Check sheet for the modelled part. Datum: model origin and axes. Units: mm. Face numbers are marked on the shaded views. A direction names the side the tool comes from. Give positions to 0.01 mm unless a question says otherwise; leave off trailing zeros. Order: outer loops, then holes, each group sorted by start corner. A loop starts at its lowest first (then second) coordinate and runs counter-clockwise, first axis right, second up. Notation, with made-up numbers: (-32.75, 76) -> (0.25, 76) arc R7 cw to (0.25, 87) -> close; hole circle Ø3 at (53, -22). An arc over 180 degrees is marked (long way). Write each question's results on one line, items separated by ' | '.
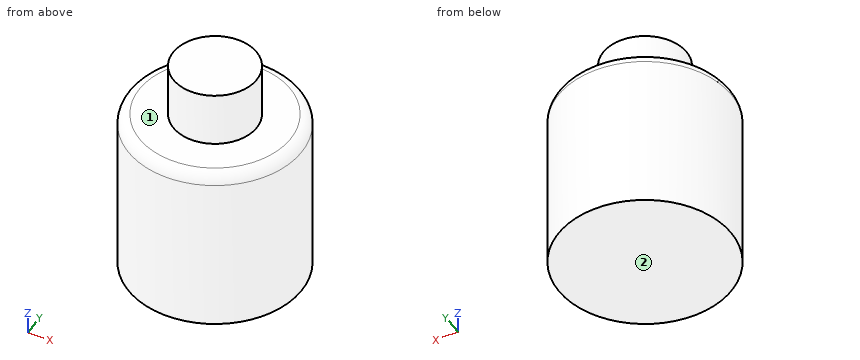
from build123d import *

# Parameters (mm, degrees)
F0_R     = 39.8272
F1_DEPTH = 78.232
F2_R     = 5.08
F3_R     = 19.201024
F4_DEPTH = 25.4


with BuildPart() as f1:
    # F0 (on Top) → F1 (new body)
    with BuildSketch(Plane.XY):
        Circle(F0_R)
    extrude(amount=F1_DEPTH)

    # F2
    f2_edges = [f1.edges().sort_by_distance(p)[0] for p in [
        (-39.8272, 0, 78.232),
    ]]
    fillet(f2_edges, radius=F2_R)

    # F3 (on face) → F4 (join)
    with BuildSketch(Plane.XY.offset(78.232)):
        Circle(F3_R)
    extrude(amount=F4_DEPTH)


solid = f1.part
1. Gauge pin test, flat ends, axial feed: pin 1 Ø3 at (y, z) = (9, 59.5) entering from -X; pin 2 Ø8 at (x, z) = (1.5, 53) entering from -Y; pin 3 Ø6 at (x, z) = (-25.5, 33) entering from -Y. Record the tip position at first contact, or that the pin passes through.
Verdict:
pin 1: stops at x = -39.11 | pin 2: stops at y = -39.83 | pin 3: stops at y = -32.86
2. Material ranges on probe 1 along Z at (x, y) = (31.5, -13); probe 2 along X at (y, z) = (1, 23.5); probe 3 along X at (y, z) = (-11.5, 92.5), recorded low to high. Write a range as from..to.
Verdict:
probe 1: z = 0..78.23 | probe 2: x = -39.81..39.81 | probe 3: x = -15.38..15.38
3. Section check A-A on x = 0. Record the cut outline in (y, z), then the cut area to 3 significant figures.
Verdict:
outline: (-39.83, 0) -> (39.83, 0) -> (39.83, 73.15) arc R5.08 ccw to (34.75, 78.23) -> (19.2, 78.23) -> (19.2, 103.63) -> (-19.2, 103.63) -> (-19.2, 78.23) -> (-34.75, 78.23) arc R5.08 ccw to (-39.83, 73.15) -> close | area: 7,200 mm^2
4. Access from +Z, -Z, +X, -X, +Y, -Y to the whole of each face (thin tool, end or side, straight path). Record for the marked faces 1 and 2.
Verdict:
face 1: +Z | face 2: -Z, +X, -X, +Y, -Y
5. Section check C-C on z = 34. Record the cut outline in (x, y), then the cut area to 3 significant figures.
Verdict:
outline: circle Ø79.65 at (0, 0) | area: 4,980 mm^2
